from build123d import *

# Parameters (mm, degrees)
SKETCH3_R           = 5.715
BOSS_EXTRUDE1_DEPTH = 10.668
SWEEP1_OUTLINE_R    = 5.715
SWEEP1_ANGLE        = 90
SKETCH9_R           = 5.715
BOSS_EXTRUDE2_DEPTH = 4.572
SKETCH11_R          = 7.3025
BOSS_EXTRUDE3_DEPTH = 14.224
FILLET1_R           = 2.54
FILLET2_R           = 2.54
SKETCH12_R          = 4.7498
CUT_EXTRUDE1_DEPTH  = 10.668
SKETCH13_R          = 6.35
CUT_EXTRUDE2_DEPTH  = 10.668


# Read off the part's stored shape, not the designer's step: Sweep1
with BuildPart() as part:
    # Sketch3 → Boss-Extrude1 (new body)
    with BuildSketch(Plane.XY):
        Circle(SKETCH3_R)
    extrude(amount=BOSS_EXTRUDE1_DEPTH)

    # Sweep1 outline → Sweep1 (revolve)
    with BuildSketch(Plane(origin=(-16.51, 0, 0), x_dir=(1, 0, 0), z_dir=(0, 0, 1))):
        with Locations((16.51, 0)):
            Circle(SWEEP1_OUTLINE_R)
    revolve(axis=Axis((-16.51, 0, 0), (0, 1, 0)), revolution_arc=SWEEP1_ANGLE)

    # Sketch9 → Boss-Extrude2 (add)
    with BuildSketch(Plane.ZY.offset(16.51)):
        with Locations(Location((-16.51, 0, 0), (0, 0, 180))):
            Circle(SKETCH9_R)
    extrude(amount=BOSS_EXTRUDE2_DEPTH)

    # Sketch11 → Boss-Extrude3 (add)
    with BuildSketch(Plane.ZY.offset(21.082)):
        with Locations((-16.51, 0)):
            Circle(SKETCH11_R)
    extrude(amount=BOSS_EXTRUDE3_DEPTH)

    # Fillet1
    # the kernel refuses this fillet: 2.54 mm, written as the material it adds along each edge
    with BuildSketch(Plane(origin=(-21.082, 0, -16.51), x_dir=(0, 0, -1), z_dir=(0, 1, 0))) as fillet1_piece_1:
        with BuildLine():
            CenterArc((8.255, -2.35464302), FILLET1_R, 112.024312837, 67.975687163)
            Line((5.715, -2.35464302), (5.6642, -2.35464302))
            Line((5.6642, -2.35464302), (5.6642, 0))
            Line((5.6642, 0), (5.715, 0.0508))
            ThreePointArc((5.715, 0.0508), (6.50875, 0.0508), (7.28345, 0.04709286))
            Line((7.28345, 0.04709286), (7.3025, 0))
        make_face()
    revolve(axis=Axis((-21.082, 0, -16.51), (-1, 0, 0)))

    # Fillet2
    fillet2_edges = [part.edges().sort_by_distance(p)[0] for p in [
        (-21.082, 7.3025, -16.51),
    ]]
    fillet(fillet2_edges, radius=FILLET2_R)

    # Sketch12 → Cut-Extrude1 (cut)
    with BuildSketch(Plane.XY.offset(10.668)):
        Circle(SKETCH12_R)
    extrude(amount=-CUT_EXTRUDE1_DEPTH, mode=Mode.SUBTRACT)

    # Sketch13 → Cut-Extrude2 (cut)
    with BuildSketch(Plane.ZY.offset(35.306)):
        with Locations((-16.51, 0)):
            Circle(SKETCH13_R)
    extrude(amount=-CUT_EXTRUDE2_DEPTH, mode=Mode.SUBTRACT)


solid = part.part
Build history of the part. All positions in model axes, mm. A direction names the side the tool comes from. Give positions to 0.01 mm unless a question says otherwise; leave off trailing zeros. Loops run counter-clockwise (first coordinate to the right, second up) from the corner with the lowest first, then second, coordinate; pieces in that order, holes last. Notation, with made-up numbers: (57, 51.5) - (69, 51.5) arc R25 ccw to (69, 81.5) - close; hole circle Ø3 at (15.5, 83). An arc over 180 degrees is marked (long way). Write item = value, one per line. Start each with the question number.
1) Drop flat-ended pins along their axis: pin 1 Ø3 at (y, z) = (0.5, -2) entering from +X; pin 2 Ø8.5 at (x, y) = (0, 0) entering from -Z; pin 3 Ø4 at (y, z) = (-2, -14.5) entering from -X. Give the stop position or say it passes through.
2) Band-saw the part on A-A on z = 4.5. Give the cut face in (x, y) (3 decimals).
3) Tool access for faces 1 (the flat face through (0, 0, 0)), 2 (the flat face through (-35.306, 7, -17)), 3 (the flat face through (-24.638, 0, -17)): list every direction of +Z, -Z, +X, -X, +Y, -Y with a clear straight run to the whole face (end or side of a thin tool).
4) Probe probe 1 along Y at (x, z) = (0, 8) (3 decimals); probe 2 along Y at (x, z) = (-28, -16.51); probe 3 along Z at (x, y) = (-30, 0.5). List the from-to ranges inside material, lowest first. Write a range as from..to.
5) Pull direction X, two halves, no side cores. Call faces 4 (the cylindrical face through (-17.6, -1.72, -21.96)), 5 (the cylindrical face through (-30.047, 1.907, -10.453)), 6 (the cylindrical face through (5.45, 1.72, 5.26)), 7 (the cylindrical face through (-3.5, 3.21, 5.41)): +X half, -X half, draft (parallel to the pull), parting line (faces both ways), or undercut.
Final values:
q1.pin_1 = 5.71
q1.pin_2 = -18.54
q1.pin_3 = -24.64
q2.outline = circle Ø11.43 at (0, 0); hole circle Ø9.5 at (0, 0)
q3.face_1 = +Z
q3.face_2 = +Z, -Z, -X, +Y, -Y
q3.face_3 = -X
q4.probe_1 = -5.715..-4.75, 4.75..5.715
q4.probe_2 = -7.3..-6.35, 6.35..7.3
q4.probe_3 = -23.8..-22.84, -10.18..-9.22
q5.face_4 = undercut
q5.face_5 = draft
q5.face_6 = parting line
q5.face_7 = undercut
